Here's how the part is built. I have some questions about the finished solid (model axes, mm). A direction names the side the tool comes from. Give positions to 0.01 mm unless a question says otherwise; leave off trailing zeros. Write each loop counter-clockwise with the first axis right and the second up, starting at its lowest first coordinate (ties: lowest second). Pieces come first, ordered by that corner, then holes. Notation, with made-up numbers: (2.25, 6) -> (7.25, 6) arc R24 ccw to (7.25, 23) -> close; hole circle Ø11 at (-13, 36.25). An arc over 180 degrees is marked (long way). Use one line per item in the form item = value.
```python
from build123d import *

# Parameters (mm, degrees)
F0_W     = 13.141317
F0_H     = 11.119574
F1_DEPTH = 17.526
F2_R     = 2.750597
F3_DEPTH = 6.35
F4_R     = 5.08


with BuildPart() as f1:
    # F0 (on Front) → F1 (new body)
    with BuildSketch(Plane.XZ):
        with Locations((-35.02122, 31.799372)):
            Rectangle(F0_W, F0_H)
    extrude(amount=F1_DEPTH)

    # F2 (on face) → F3 (cut)
    with BuildSketch(Plane.XY.offset(37.359159)):
        with Locations((-37.022505, -8.269278)):
            Circle(F2_R)
    extrude(amount=-F3_DEPTH, mode=Mode.SUBTRACT)

    # F4
    f4_edges = [f1.edges().sort_by_distance(p)[0] for p in [
        (-28.450562, -8.763, 37.359159),
        (-41.591879, -8.763, 26.239585),
    ]]
    fillet(f4_edges, radius=F4_R)


solid = f1.part
```
Q1. I want a section at C-C, the plane y = -6.5. Write out the boundary of the cut face in (x, z), and give its area (3 significant figures).
Result set:
outline = (-41.59, 31.32) arc R5.08 ccw to (-36.51, 26.24) -> (-28.45, 26.24) -> (-28.45, 32.28) arc R5.08 ccw to (-33.53, 37.36) -> (-34.92, 37.36) -> (-34.92, 31.01) -> (-39.13, 31.01) -> (-39.13, 37.36) -> (-41.59, 37.36) -> close
area = 108 mm2
Q2. Which directions (+Z, -Z, +X, -X, +Y, -Y) give clear straight access to the entire face, cutting with the end or side of a thin tool? Please do faces 4 (the face through (-39, -11, 37.359)), 5 (the face through (-37, -8, 31.009)).
Result set:
face_4 = +Z, +X, -X, +Y, -Y
face_5 = +Z
Q3. If we mould it in two halves opening along Y, with no side actions, what happens to faces 1 (the face through (-40.143, -8.886, 27.767)), 2 (the face through (-39.77, -8.15, 34.23)), 3 (the face through (-35, 0, 32))? For each: +Y half, -Y half, draft (parallel to the pull), parting line (faces both ways), or undercut.
Result set:
face_1 = draft
face_2 = undercut
face_3 = +Y half
Q4. Will this pin go through, and if not, where does the flat tip stop? pin 1 Ø1 at (x, y) = (-31, -13) entering from +Z.
Result set:
pin_1 = 36.94
Q5. I want a section at B-B, the plane x = -34.5. Write out the boundary of the cut face in (y, z), and give its area (3 significant figures).
Result set:
outline = (-17.53, 26.24) -> (0, 26.24) -> (0, 37.36) -> (-7.17, 37.36) -> (-7.17, 31.01) -> (-9.37, 31.01) -> (-9.37, 37.36) -> (-17.53, 37.36) -> close
area = 181 mm2
Q6. If I drill on line 1 along Z through (x, y) = (-35.5, -8.75); line 2 along X through (y, z) = (-6.5, 32); line 3 along X through (y, z) = (-6, 34.5), over which ranges is the centre line in solid material (lowest first)? Write a range as from..to.
Result set:
line_1 = 26.24..31.01
line_2 = -41.59..-39.13, -34.92..-28.45
line_3 = -41.59..-38.58, -35.47..-28.96
Q7. I want a section at A-A, the plane z = 33.5. Write out the boundary of the cut face in (x, y), and give its area (3 significant figures).
Result set:
outline = (-41.59, -17.53) -> (-28.6, -17.53) -> (-28.6, 0) -> (-41.59, 0) -> close; hole circle Ø5.5 at (-37.02, -8.27)
area = 204 mm2
Q8. I want a section at D-D, the plane y = -14.75. Write out the boundary of the cut face in (x, z), and give its area (3 significant figures).
Result set:
outline = (-41.59, 31.32) arc R5.08 ccw to (-36.51, 26.24) -> (-28.45, 26.24) -> (-28.45, 32.28) arc R5.08 ccw to (-33.53, 37.36) -> (-41.59, 37.36) -> close
area = 135 mm2
